Autodesk Inventor part; units mm, degrees
ref_plane "YZ Plane" through (0, 0, 0) normal (1, 0, 0) x (0, 1, 0)
ref_plane "XZ Plane" through (0, 0, 0) normal (0, 1, 0) x (-1, 0, 0)
ref_plane "XY Plane" through (0, 0, 0) normal (0, 0, 1) x (1, 0, 0)
sketch "T-Slot 4040 Base" plane through (0, 0, 0) normal (0, 0, 1) x (1, 0, 0)
  line L0 (-28, 0) -> (28, 0) construction
  line L1 (0, -28) -> (0, 28) construction
  circle A0 centre (0, 0) radius 3.4
  line L2 (-7.5, -7.5) -> (7.5, -7.5)
  line L3 (7.5, -7.5) -> (7.5, 7.5)
  line L4 (7.5, 7.5) -> (-7.5, 7.5)
  line L5 (-7.5, 7.5) -> (-7.5, -7.5)
  line L6 (-7.5, -7.5) -> (7.5, 7.5) construction
  line L7 (7.5, -7.5) -> (-7.5, 7.5) construction
  line L8 (20, 4) -> (15.5, 4)
  line L9 (15.5, 4) -> (15.5, 12)
  line L10 (15.5, 12) -> (7.5, 4)
  line L11 (4, 20) -> (4, 15.5)
  line L12 (4, 15.5) -> (12, 15.5)
  line L13 (12, 15.5) -> (4, 7.5)
  line L14 (7.5, -7.5) -> (-7.5, -7.5)
  arc A1 (15.5, 9.5858) -> (13.7929, 10.2929) centre (14.5, 9.5858) ccw
  arc A2 (10.2929, 13.7929) -> (9.5858, 15.5) centre (9.5858, 14.5) ccw
  line L15 (-20, 20) -> (20, 20)
  line L16 (20, 20) -> (20, -20)
  line L17 (20, -20) -> (-20, -20)
  line L18 (-20, -20) -> (-20, 20)
  line L19 (-20, 20) -> (20, -20) construction
  line L20 (20, 20) -> (-20, -20) construction
  line L21 (-4, 15.5) -> (-12, 15.5)
  arc A3 (-9.5858, 15.5) -> (-10.2929, 13.7929) centre (-9.5858, 14.5) ccw
  line L22 (-12, 15.5) -> (-4, 7.5)
  line L23 (-15.5, 12) -> (-7.5, 4)
  line L24 (-20, 4) -> (-15.5, 4)
  arc A4 (-13.7929, 10.2929) -> (-15.5, 9.5858) centre (-14.5, 9.5858) ccw
  line L25 (-15.5, 4) -> (-15.5, 12)
  line L26 (-4, 20) -> (-4, 15.5)
  line L27 (-15.5, -4) -> (-15.5, -12)
  arc A5 (-15.5, -9.5858) -> (-13.7929, -10.2929) centre (-14.5, -9.5858) ccw
  line L28 (-15.5, -12) -> (-7.5, -4)
  line L29 (-12, -15.5) -> (-4, -7.5)
  line L30 (-4, -20) -> (-4, -15.5)
  arc A6 (-10.2929, -13.7929) -> (-9.5858, -15.5) centre (-9.5858, -14.5) ccw
  line L31 (-4, -15.5) -> (-12, -15.5)
  line L32 (-20, -4) -> (-15.5, -4)
  line L33 (4, -15.5) -> (12, -15.5)
  arc A7 (9.5858, -15.5) -> (10.2929, -13.7929) centre (9.5858, -14.5) ccw
  line L34 (12, -15.5) -> (4, -7.5)
  line L35 (15.5, -12) -> (7.5, -4)
  line L36 (20, -4) -> (15.5, -4)
  arc A8 (13.7929, -10.2929) -> (15.5, -9.5858) centre (14.5, -9.5858) ccw
  line L37 (15.5, -4) -> (15.5, -12)
  line L38 (4, -20) -> (4, -15.5)
  point P0 (4.9274, 7.75)
  point P1 (9.5858, 15.5)
  point P2 (-20, 20)
  point P3 (-7.5, -7.5)
  point P4 (-20, -20)
  point P5 (7.5, -7.5)
  point P6 (20, -20)
  point P7 (-9.5858, -15.5)
  point P8 (-4, -7.5)
  point P9 (15.5, -9.5858)
  point P10 (7.5, -4)
  point P11 (-15.5, 9.5858)
  point P12 (-4, 7.5)
  dimension "d35" = 6.8
  dimension "d37" = 12
  dimension "d38" = 1
  dimension "d43" = 40
  dimension "d44" = 40
  dimension "d45" = 4.5
  dimension "d46" = 4
  dimension "d53" = 360
extrude "Extrusion1" add sketch "T-Slot 4040 Base" along normal blind 1500 contours L5 L4 L3 L2 | L2 L29 L31 L30 L17 L18 L32 L27 L28 L5 | L2 L3 L35 L37 L36 L16 L17 L38 L33 L34 | A6 L31 L29 | L23 L25 L24 L18 L15 L26 L21 L22 L4 L5 | L28 L27 A5 | L34 L33 A7 | A4 L25 L23 | L3 L4 L13 L12 L11 L15 L16 L8 L9 L10 | A8 L37 L35 | L22 L21 A3 | L10 L9 A1 | A2 L12 L13
fillet "Rundung1" radius 1 16 edges at (4, 15.5, 750) (15.5, 4, 750) (20, 4, 750) (4, 20, 750) (-20, 4, 750) (-15.5, 4, 750) (-4, 15.5, 750) (-4, 20, 750) (-4, -15.5, 750) (-4, -20, 750) (4, -15.5, 750) (4, -20, 750) (15.5, -4, 750) (20, -4, 750) (-20, -4, 750) (-15.5, -4, 750)
fillet "Rundung2" radius 4 12 edges at (4, 7.5, 750) (7.5, 4, 750) (-20, 20, 750) (-20, -20, 750) (20, 20, 750) (20, -20, 750) (7.5, -4, 750) (-7.5, -4, 750) (-7.5, 4, 750) (4, -7.5, 750) (-4, -7.5, 750) (-4, 7.5, 750)
properties part number "T-SLOT 4040 B-Type 1500mm"
Check sheet for the modelled part. Datum: model origin and axes. Units: mm. Round coordinates to 2 decimals unless told otherwise and drop trailing zeros. Write item = value, one per line. Start each with the question number.
1) Release check for a two-part mould opening along Z. For faces 1 (the flat face through (4, 0, 0)), 2 (the flat face through (4, 0, 1500)) record: released by +Z, released by -Z, zero draft, split by the parting line, or undercut.
2) Thickness scan on probe 1 along Y at (x, z) = (6, 714.5); probe 2 along X at (y, z) = (5, 336); probe 3 along Y at (x, z) = (-7, 399). Record the ranges inside material, lowest first.
3) Gauge pin test, flat ends, axial feed: pin 1 Ø2 at (y, z) = (-18, 844) entering from -X; pin 2 Ø5 at (x, z) = (4.5, 893.5) entering from +Y; pin 3 Ø1.4 at (x, z) = (0, 932) entering from +Y; pin 4 Ø3 at (x, z) = (18.5, 1082) entering from -Y. Record the tip position at first contact, or that the pin passes through.
Results are:
q1.face_1 = released by -Z
q1.face_2 = released by +Z
q2.probe_1 = -20 to -15.5, -9.5 to 9.5, 15.5 to 20
q2.probe_2 = -20 to -15.5, -8.51 to 8.51, 15.5 to 20
q2.probe_3 = -20 to -15.5, -10.5 to 10.5, 15.5 to 20
q3.pin_1 = -19.87
q3.pin_2 = 20
q3.pin_3 = 7.5
q3.pin_4 = -19.87
